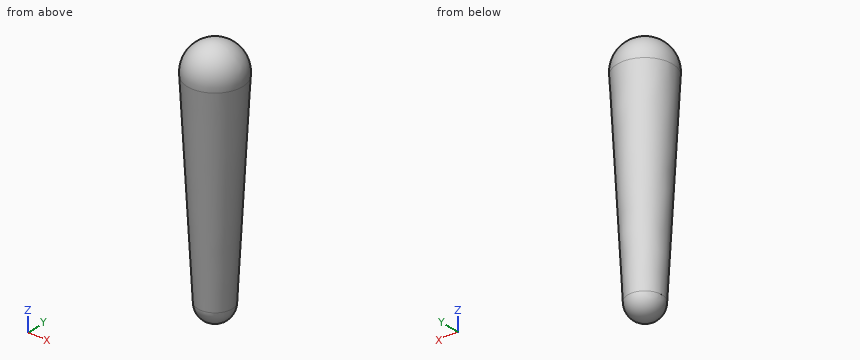
```python
from build123d import *

# Parameters (mm, degrees)
SKETCH1_R           = 57.15
BOSS_EXTRUDE1_DEPTH = 419.1
BOSS_EXTRUDE1_DRAFT = -3


# Read off the part's stored shape, not the designer's step: Revolve2
with BuildPart() as part:
    # Sketch1 → Boss-Extrude1 (with draft: the straight prism first)
    with BuildSketch(Plane.XY):
        Circle(SKETCH1_R)
    extrude(amount=-BOSS_EXTRUDE1_DEPTH)
    # Boss-Extrude1: the draft: its side faces are tilted about the plane it starts from
    boss_extrude1_sides = [part.faces().sort_by_distance(p)[0] for p in [
        (-57.15, 0, -209.55),
    ]]
    draft(boss_extrude1_sides, Plane.XY, BOSS_EXTRUDE1_DRAFT)

    # Sketch4 → Revolve1 (revolve)
    with BuildSketch(Plane(origin=(0, 0, 0), x_dir=(0, 0, -1), z_dir=(1, 0, 0))):
        with BuildLine():
            Line((419.1, 35.185899702), (419.1, -35.185899702))
            ThreePointArc((419.1, -35.185899702), (454.285899702, 0), (419.1, 35.185899702))
        make_face()
    revolve(axis=Axis((0, 35.185899702, -419.1), (0, -1, 0)))

    # Revolve2 outline → Revolve2 (revolve)
    with BuildSketch(Plane.XZ):
        with BuildLine():
            Line((56.836926314, 0), (56.836926314, -5.973801733))
            ThreePointArc((56.836926314, -5.973801733), (42.470726795, 38.240814132), (0, 57.15))
            Line((0, 57.15), (0, 0))
            Line((0, 0), (56.836926314, 0))
        make_face()
    revolve(axis=Axis((0, 0, 0), (0, 0, 1)))


solid = part.part
```
CAD build for the part. Positions are in the model's coordinates, mm. Round coordinates to 2 decimals unless told otherwise and drop trailing zeros. Loops run counter-clockwise (first coordinate to the right, second up) from the corner with the lowest first, then second, coordinate; pieces in that order, holes last. Notation, with made-up numbers: M -32.75,62.25 L 9.25,62.25 A30 ccw 9.25,94.25 Z; hole C 20.5,12 d9. An arc over 180 degrees is marked long. Use a Markdown table: item, result. Add a question column.
(1) Flat gauge pins, fed straight in: pin 1 (6 mm diameter, centred on x = 5, z = -152, fed in from +Y); pin 2 (10 mm diameter, centred on x = 14, y = -32, fed in from -Z); pin 3 (1 mm diameter, centred on y = 38.5, z = -68.5, fed in from +X). Where does each tip first touch, or does it go through?
(2) Cut at C-C (z = -326.5). Give the cut face in (x, y), and give its area (3 significant figures).
(3) Drill centre lines: line 1 (X direction, y = 8, z = -211.5); line 2 (Y direction, x = 7.5, z = -72); line 3 (X direction, y = -8, z = -35.5). Where is each one in solid material? Low to high.
(4) Cut at D-D (z = -55.5). Give the cut face in (x, y), and give its area (3 significant figures).
(5) Cut at A-A (x = 0). Give the cut face in (y, z).
Geometry says:
| question | item | result |
|---|---|---|
| 1 | pin 1 | stops at y = 49.21 |
| 1 | pin 2 | stops at z = -437.6 |
| 1 | pin 3 | stops at x = 37.75 |
| 2 | outline | C 0,0 d80.08 |
| 2 | area | 5,040 mm² |
| 3 | line 1 | x = -45.37 to 45.37 |
| 3 | line 2 | y = -52.85 to 52.85 |
| 3 | line 3 | x = -54.71 to 54.71 |
| 4 | outline | C 0,0 d108.48 |
| 4 | area | 9,240 mm² |
| 5 | outline | M -56.84,-5.97 L -35.19,-419.1 A35.19 ccw 35.19,-419.1 L 56.84,-5.97 A57.15 ccw long Z |
